For this review, take the finished solid that the model builds, in its own axes (mm). Coordinates: 2 decimals unless noted, no trailing zeros. Loops run counter-clockwise (first coordinate to the right, second up) from the corner with the lowest first, then second, coordinate; pieces in that order, holes last. Notation, with made-up numbers: M 23,64 L 47,64 A15 ccw 47,92 Z; hole C 79,-30 d11. An arc over 180 degrees is marked long. Put each result on its own line as item: value.
Autodesk Inventor part; units mm, degrees
ref_plane "Work Plane1" through (48, 48, 0) normal (0.7071, -0.7071, 0) x (0.7071, 0.7071, 0)
ref_plane "YZ Plane" through (0, 0, 0) normal (1, 0, 0) x (0, 1, 0)
ref_plane "XZ Plane" through (0, 0, 0) normal (0, 1, 0) x (-1, 0, 0)
sketch "Sketch1" plane through (0, 0, 0) normal (0, 0, 1) x (1, 0, 0)
  line L0 (-41.5, 58) -> (41.5, 58)
  line L1 (41.5, 58) -> (41.5, 158)
  line L2 (41.5, 158) -> (-41.5, 158)
  line L3 (-41.5, 158) -> (-41.5, 58)
  line L4 (58, 41.5) -> (158, 41.5)
  line L5 (158, 41.5) -> (158, -41.5)
  line L6 (158, -41.5) -> (58, -41.5)
  line L7 (58, -41.5) -> (58, 41.5)
  line L8 (-131.1952, 0) -> (204.4844, 0) construction
  line L9 (-48, 48) -> (48, 48)
  line L10 (48, 48) -> (48, -48)
  line L11 (48, -48) -> (-48, -48)
  line L12 (-48, -48) -> (-48, 48)
  line L13 (0, 180.9439) -> (0, -136.3054) construction
  point P0 (0, 0)
  point P1 (-48, 0)
  point P2 (0, 48)
  point P3 (0, 58)
  point P4 (58, 0)
  dimension "d0" = 83
  dimension "d1" = 100
  dimension "d2" = 100
  dimension "d3" = 83
  dimension "d5" = 96
  dimension "d6" = 96
  dimension "d7" = 10
  dimension "d8" = 10
sketch "Sketch2" plane through (0, 0, 0) normal (0, 0, 1) x (1, 0, 0)
  line L0 (41.5, 158) -> (-41.5, 158)
  line L1 (41.5, 58) -> (41.5, 158)
  line L2 (-48, 48) -> (48, 48)
  line L3 (48, 48) -> (48, -48)
  line L4 (58, -41.5) -> (58, 41.5)
  line L5 (58, 41.5) -> (158, 41.5)
  line L6 (-41.5, 58) -> (41.5, 58)
  line L7 (158, 41.5) -> (158, -41.5)
  line L8 (48, 48) -> (136.7868, 136.7868) construction
  line L9 (35.5, 78) -> (57.5, 78)
  line L10 (57.5, 78) -> (57.5, 138)
  line L11 (57.5, 138) -> (35.5, 138)
  line L12 (35.5, 138) -> (35.5, 78)
  line L13 (41.5, 108) -> (-41.5, 108) construction
  line L14 (108, 41.5) -> (108, -41.5) construction
  line L15 (41.5, 158) -> (220.1006, 158) construction
  line L16 (158, 41.5) -> (158, 206.0131) construction
  line L17 (115.5736, 158) -> (158, 115.5736) construction
  line L18 (41.5, 138) -> (41.5, 78) construction
  line L19 (51.5, 138) -> (51.5, 78) construction
  line L20 (46.5, 138) -> (46.5, 78) construction
  line L21 (51.5, 158) -> (51.5, 70.6421)
  line L22 (60.0355, 67.1066) -> (133.2513, 140.3223)
  arc A0 (51.5, 158) -> (133.2513, 140.3223) centre (109.2071, 226.9991) ccw
  line L23 (68.9045, 84.4609) -> (84.4609, 68.9045)
  line L24 (84.4609, 68.9045) -> (126.8873, 111.331)
  line L25 (126.8873, 111.331) -> (111.331, 126.8873)
  line L26 (111.331, 126.8873) -> (68.9045, 84.4609)
  line L27 (80.2183, 73.1472) -> (122.6447, 115.5736) construction
  line L28 (105.6741, 90.1177) -> (90.1177, 105.6741) construction
  line L29 (73.1472, 80.2183) -> (115.5736, 122.6447) construction
  line L30 (76.6827, 76.6827) -> (119.1091, 119.1091) construction
  circle A1 centre (73.1472, 84.4609) radius 2.25
  circle A2 centre (111.331, 122.6447) radius 2.25
  circle A3 centre (84.4609, 73.1472) radius 2.25
  circle A4 centre (122.6447, 111.331) radius 2.25
  circle A5 centre (38.5, 135) radius 2.25
  circle A6 centre (38.5, 81) radius 2.25
  circle A7 centre (54.5, 135) radius 2.25
  circle A8 centre (54.5, 81) radius 2.25
  arc A9 (51.5, 70.6421) -> (60.0355, 67.1066) centre (56.5, 70.6421) ccw
  circle A10 centre (56.5, 70.6421) radius 2.25
  point P0 (0, 0)
  point P1 (158, 158)
  dimension "d23" = 30
  dimension "d25" = 45
  dimension "d30" = 10
  dimension "d37" = 10
  dimension "d38" = 60
  dimension "d39" = 4.5
  dimension "d40" = 3
  dimension "d42" = 4.5
  dimension "d43" = 3
  dimension "d46" = 60
  dimension "d47" = 30
  dimension "d48" = 4.5
  dimension "d49" = 3
  dimension "d50" = 3
  dimension "d51" = 4.5
  dimension "d52" = 3
  dimension "d53" = 3
  dimension "d54" = 5
  dimension "d55" = 25
  dimension "d57" = 3
  dimension "d58" = 3
  dimension "d59" = 3
  dimension "d60" = 3
  dimension "d77" = 4.5
ref_plane "Work Plane1" through (48, 48, 0) normal (0.7071, -0.7071, 0) x (0.7071, 0.7071, 0)
extrude "Extrusion7" add sketch "Sketch2" along normal blind 1 contours L21 L11 L10 L9 | L9 L10 L11 L21 A0 L22 L25 L26 L23 A9 | L23 L26 L25 L22 | A1 | A8
properties part number "SolarFolds_Sketch"
(1) Draft analysis for pull direction Y (two halves, no side actions). For faces 1 (the flat face through (74, 112, 0)), 2 (the cylindrical face through (52.714, 136.369, 0.493)), 3 (the cylindrical face through (54.663, 65.992, 0.493)), state which applies: +Y half, -Y half, draft (parallel to the pull), parting line (faces both ways), or undercut.
Determined:
face 1: draft
face 2: undercut
face 3: -Y half
(2) Add section D-D (y = 98.5). Write out the cut boundary in (x, z).
Determined:
outline: M 51.5,0 L 91.43,0 L 91.43,1 L 51.5,1 Z
(3) Wall thickness on line 1 along Y through (x, z) = (56.5, 0.85); line 2 along Y through (x, z) = (56, 0.5); line 3 along X through (y, z) = (135, 0.5): over which ranges is each line inside the solid? List them lowest first. Write a range as [from, to].
Determined:
line 1: y = [65.64, 68.39], [72.89, 133.97], [136.03, 154.11]
line 2: y = [65.67, 68.45], [72.84, 133.32], [136.68, 154.47]
line 3: x = [51.5, 52.25], [56.75, 127.93]
(4) Add section C-C (z = 0.15). Write out the cut boundary in (x, y), plus the area to 3 significant figures.
Determined:
outline: M 51.5,70.64 A5 ccw 60.04,67.11 L 133.25,140.32 A89.95 cw 51.5,158 Z; hole C 54.5,135 d4.5; hole C 56.5,70.64 d4.5; hole C 111.33,122.64 d4.5
area: 3,400 mm^2
(5) Add section B-B (y = 135). Write out the cut boundary in (x, z), plus the area to 3 significant figures.
Determined:
outline: M 51.5,0 L 52.25,0 L 52.25,1 L 51.5,1 Z; M 56.75,0 L 127.93,0 L 127.93,1 L 56.75,1 Z
area: 71.9 mm^2
(6) For pin 1 (4 mm diameter, centred on x = 56.5, y = 70.64, fed in from +Z), flat-tipped, find the tip position at first contact; note if it passes through.
Determined:
pin 1: passes through
(7) Add section A-A (x = 111.5). Write out the cut boundary in (y, z).
Determined:
outline: M 118.57,0 L 120.4,0 L 120.4,1 L 118.57,1 Z; M 124.89,0 L 137.08,0 L 137.08,1 L 124.89,1 Z
